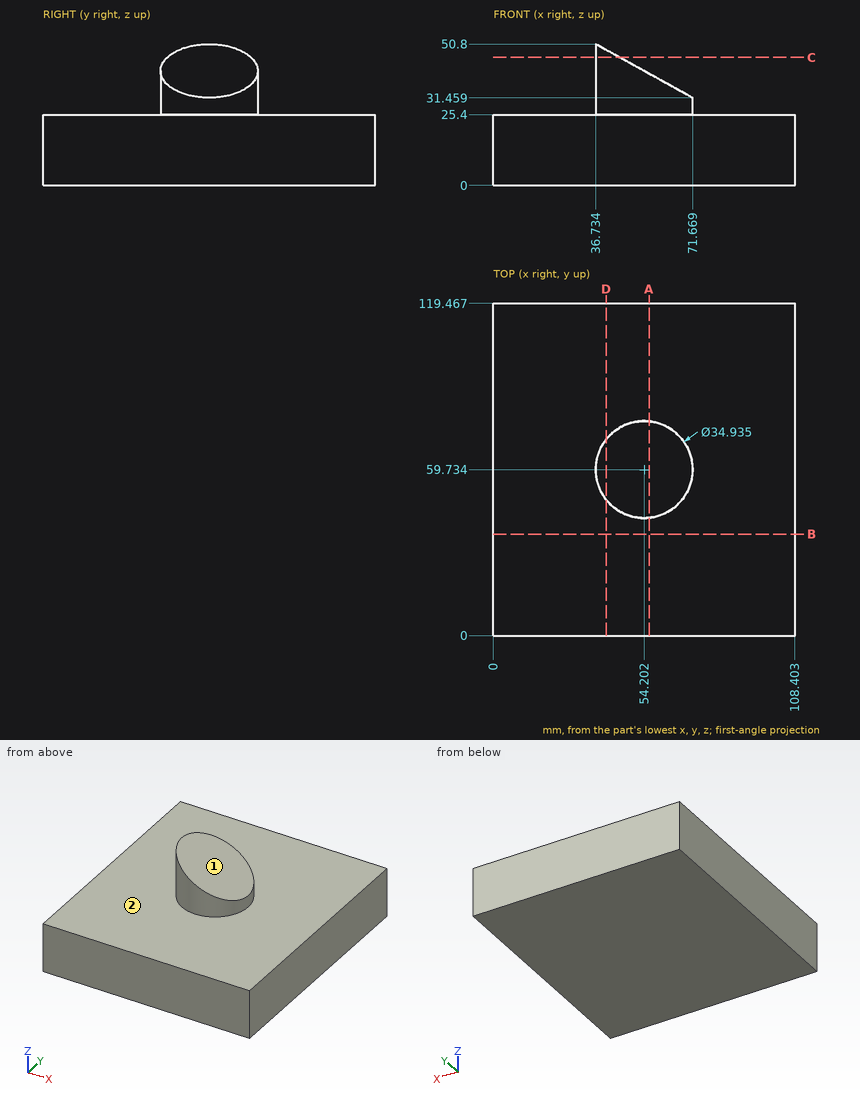
The drawing under review shows one solid part. Ordinate dimensions are in mm from its lowest x, y, z. A direction names the side the tool comes from. Round coordinates to 2 decimals unless told otherwise and drop trailing zeros. Loops run counter-clockwise (first coordinate to the right, second up) from the corner with the lowest first, then second, coordinate; pieces in that order, holes last. Notation, with made-up numbers: (59, 13) -> (107, 13) arc R23 ccw to (107, 34) -> close; hole circle Ø10 at (5.25, -37.5). An arc over 180 degrees is marked (long way). Answer in a Markdown table with one row per item.
1) For pin 1 Ø1 at (x, y) = (88, 16.5) entering from +Z, flat-tipped, find the tip position at first contact; note if it passes through.
Taken from the geometry:
| item | result |
|---|---|
| pin 1 | stops at z = 25.4 |
2) Consider section D-D, the plane x = 40.5. Write out the cut boundary in (y, z) (1 decimal).
Taken from the geometry:
| item | result |
|---|---|
| outline | (0, 0) -> (119.5, 0) -> (119.5, 25.4) -> (70.6, 25.4) -> (70.6, 48.7) -> (48.9, 48.7) -> (48.9, 25.4) -> (0, 25.4) -> close |
3) Consider section C-C, the plane z = 46. Write out the cut boundary in (x, y) (1 decimal).
Taken from the geometry:
| item | result |
|---|---|
| outline | (45.4, 44.6) -> (45.4, 74.8) arc R17.5 ccw to start |
4) Consider section A-A, the plane x = 56. Write out the cut boundary in (y, z), plus the area to 3 significant figures.
Taken from the geometry:
| item | result |
|---|---|
| outline | (0, 0) -> (119.47, 0) -> (119.47, 25.4) -> (77.11, 25.4) -> (77.11, 40.13) -> (42.36, 40.13) -> (42.36, 25.4) -> (0, 25.4) -> close |
| area | 3,550 mm² |
5) Consider section B-B, the plane y = 36.5. Write out the cut boundary in (x, z), plus the area to 3 significant figures.
Taken from the geometry:
| item | result |
|---|---|
| outline | (0, 0) -> (108.4, 0) -> (108.4, 25.4) -> (0, 25.4) -> close |
| area | 2,750 mm² |
6) Tool access review of the marked faces 1 and 2: name each direction out of +Z, -Z, +X, -X, +Y, -Y from which nothing blocks a thin tool from reaching the whole face with its end or side.
Taken from the geometry:
| item | result |
|---|---|
| face 1 | +Z, +X, +Y, -Y |
| face 2 | +Z |
7) Wall thickness on line 1 along Z through (x, y) = (86.5, 14); line 2 along Y through (x, z) = (42, 40.5) (1 decimal); line 3 along Y through (x, z) = (43.5, 47): over which ranges is each line inside the solid? List them lowest first.
Taken from the geometry:
| item | result |
|---|---|
| line 1 | z = 0 to 25.4 |
| line 2 | y = 47.2 to 72.2 |
| line 3 | y = 45.93 to 73.54 |
